from build123d import *

# Parameters (mm, degrees)
SKETCH1_W               = 80
SKETCH1_H               = 13
BOSS_EXTRUDE1_DEPTH     = 13
CUT_EXTRUDE1_DEPTH      = 7.5
CUT_EXTRUDE1_DEPTH_BACK = 7.5
CUT_EXTRUDE2_REACH      = 15
SKETCH4_R               = 1.5


with BuildPart() as part:
    # Sketch1 → Boss-Extrude1 (new body)
    with BuildSketch(Plane(origin=(0, 0, 0), x_dir=(1, 0, 0), z_dir=(0, 1, 0))):
        Rectangle(SKETCH1_W, SKETCH1_H)
    extrude(amount=BOSS_EXTRUDE1_DEPTH)

    # Sketch3 → Cut-Extrude1 (cut, two sides)
    with BuildSketch(Plane.XY) as cut_extrude1_sk:
        with BuildLine():
            ThreePointArc((0, 2.5), (8, 6.5), (0, 10.5))
            ThreePointArc((0, 10.5), (-8, 6.5), (0, 2.5))
        make_face()
    extrude(amount=CUT_EXTRUDE1_DEPTH, mode=Mode.SUBTRACT)
    extrude(cut_extrude1_sk.sketch, amount=-CUT_EXTRUDE1_DEPTH_BACK, mode=Mode.SUBTRACT)

    # Sketch4 → Cut-Extrude2 (cut, up to next)
    with BuildSketch(Plane(origin=(0, 13, 0), x_dir=(1, 0, 0), z_dir=(0, 1, 0)), mode=Mode.PRIVATE) as cut_extrude2_sk1:
        with Locations((-35, 0)):
            Circle(SKETCH4_R)
    cut_extrude2_tool1 = extrude(cut_extrude2_sk1.sketch, amount=-CUT_EXTRUDE2_REACH, mode=Mode.PRIVATE) & part.part
    add(cut_extrude2_tool1.solids().sort_by_distance((-35, 13, 0))[0], mode=Mode.SUBTRACT)
    # Sketch4 → Cut-Extrude2 (cut, up to next)
    with BuildSketch(Plane(origin=(0, 13, 0), x_dir=(1, 0, 0), z_dir=(0, 1, 0)), mode=Mode.PRIVATE) as cut_extrude2_sk2:
        with Locations((-20, 0)):
            Circle(SKETCH4_R)
    cut_extrude2_tool2 = extrude(cut_extrude2_sk2.sketch, amount=-CUT_EXTRUDE2_REACH, mode=Mode.PRIVATE) & part.part
    add(cut_extrude2_tool2.solids().sort_by_distance((-20, 13, 0))[0], mode=Mode.SUBTRACT)
    # Sketch4 → Cut-Extrude2 (cut, up to next)
    with BuildSketch(Plane(origin=(0, 13, 0), x_dir=(1, 0, 0), z_dir=(0, 1, 0)), mode=Mode.PRIVATE) as cut_extrude2_sk3:
        with Locations((20, 0)):
            Circle(SKETCH4_R)
    cut_extrude2_tool3 = extrude(cut_extrude2_sk3.sketch, amount=-CUT_EXTRUDE2_REACH, mode=Mode.PRIVATE) & part.part
    add(cut_extrude2_tool3.solids().sort_by_distance((20, 13, 0))[0], mode=Mode.SUBTRACT)
    # Sketch4 → Cut-Extrude2 (cut, up to next)
    with BuildSketch(Plane(origin=(0, 13, 0), x_dir=(1, 0, 0), z_dir=(0, 1, 0)), mode=Mode.PRIVATE) as cut_extrude2_sk4:
        with Locations((35, 0)):
            Circle(SKETCH4_R)
    cut_extrude2_tool4 = extrude(cut_extrude2_sk4.sketch, amount=-CUT_EXTRUDE2_REACH, mode=Mode.PRIVATE) & part.part
    add(cut_extrude2_tool4.solids().sort_by_distance((35, 13, 0))[0], mode=Mode.SUBTRACT)


solid = part.part
Geometry check sheet. Reference: the model listing, model coordinates, mm. Give positions to 0.01 mm unless a question says otherwise; leave off trailing zeros. Order: outer loops, then holes, each group sorted by start corner. A loop starts at its lowest first (then second) coordinate and runs counter-clockwise, first axis right, second up.
1) Cross-section at D-D (z = -3.5). Record the boundary of the cut face in (x, y).
Results are:
outline: (-40, 0) - (40, 0) - (40, 13) - (-40, 13) - close; hole (0, 2.5) arc R5 ccw (long way) to (0, 10.5) arc R5 ccw (long way) to start
2) Cross-section at C-C (x = 7). Record the boundary of the cut face in (y, z).
Results are:
outline: (0, -6.5) - (3.5, -6.5) - (3.5, 6.5) - (0, 6.5) - close; (9.5, -6.5) - (13, -6.5) - (13, 6.5) - (9.5, 6.5) - close
3) Cross-section at A-A (y = 6.5). Record the boundary of the cut face in (x, z).
Results are:
outline: (-40, -6.5) - (-8, -6.5) - (-8, 6.5) - (-40, 6.5) - close; (8, -6.5) - (40, -6.5) - (40, 6.5) - (8, 6.5) - close; hole circle Ø3 at (-35, 0); hole circle Ø3 at (-20, 0); hole circle Ø3 at (20, 0); hole circle Ø3 at (35, 0)
4) Draft check along Y on faces 1 (the flat face through (-1, 0, 0)), 2 (the cylindrical face through (7.998, 6.345, -0.091)), 3 (the flat face through (40, 6, 0)), 4 (the cylindrical face through (-7.998, 6.655, -0.091)). Enter one of: released by +Y, released by -Y, zero draft, split by the parting line, or undercut.
Results are:
face 1: released by -Y
face 2: undercut
face 3: zero draft
face 4: undercut
5) Cross-section at B-B (z = 0). Record the boundary of the cut face in (x, y), then the cut area to 3 significant figures.
Results are:
outline: (-40, 0) - (-36.5, 0) - (-36.5, 13) - (-40, 13) - close; (-33.5, 0) - (-21.5, 0) - (-21.5, 13) - (-33.5, 13) - close; (-18.5, 0) - (18.5, 0) - (18.5, 13) - (-18.5, 13) - close; (21.5, 0) - (33.5, 0) - (33.5, 13) - (21.5, 13) - close; (36.5, 0) - (40, 0) - (40, 13) - (36.5, 13) - close; hole (0, 2.5) arc R5 ccw (long way) to (0, 10.5) arc R5 ccw (long way) to start
area: 749 mm2
6) Material ranges on probe 1 along Z at (x, y) = (-20, 8.75); probe 2 along X at (y, z) = (7, 0); probe 3 along X at (y, z) = (0.5, -0.5), recorded low to high.
Results are:
probe 1: z = -6.5 to -1.5, 1.5 to 6.5
probe 2: x = -40 to -36.5, -33.5 to -21.5, -18.5 to -7.97, 7.97 to 18.5, 21.5 to 33.5, 36.5 to 40
probe 3: x = -40 to -36.41, -33.59 to -21.41, -18.59 to 18.59, 21.41 to 33.59, 36.41 to 40
